Here's the drawing with two shaded views (mm, measured from the low corner). I have some questions. A direction names the side the tool comes from. Give positions to 0.01 mm unless a question says otherwise; leave off trailing zeros. Write each loop counter-clockwise with the first axis right and the second up, starting at its lowest first coordinate (ties: lowest second). Pieces come first, ordered by that corner, then holes.
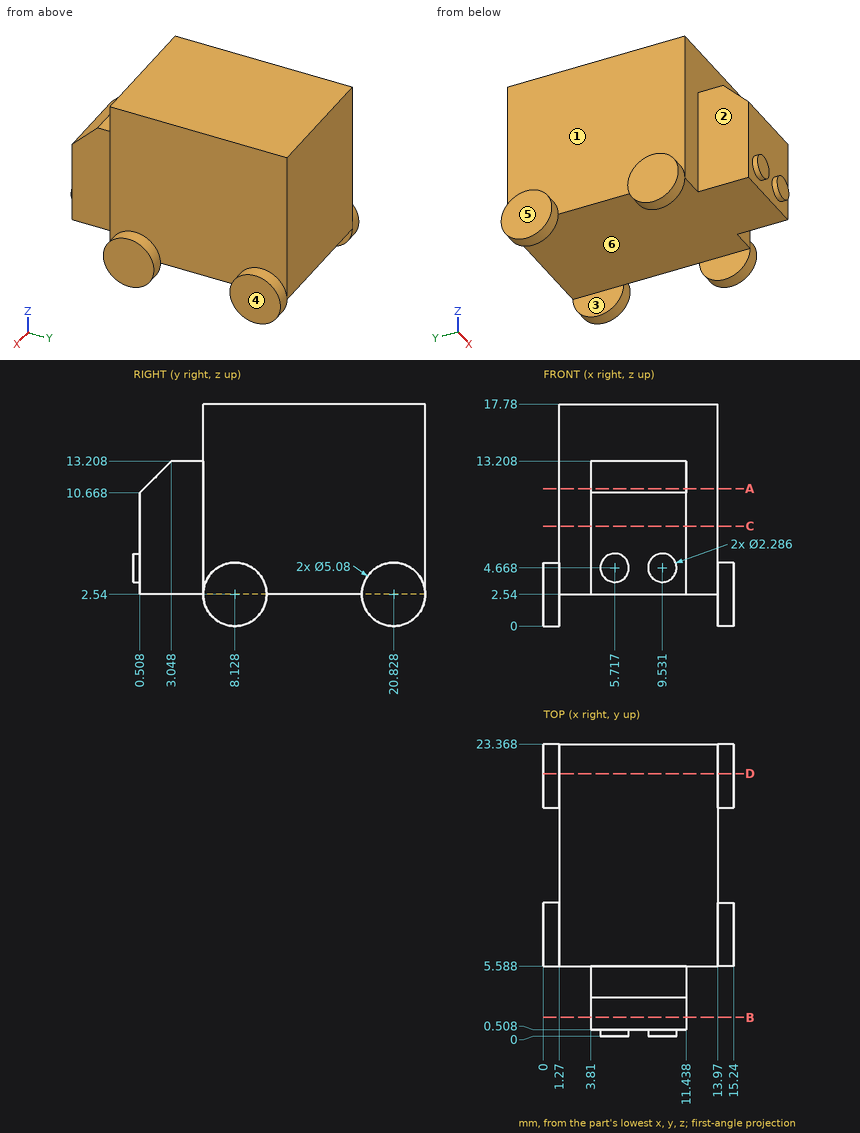
(1) Imagine slicing it at B-B, the plane y = 1.5. Write out the boundary of the cut face in (x, z).
Returned:
outline: (3.81, 2.54) - (11.44, 2.54) - (11.44, 11.66) - (3.81, 11.66) - close
(2) For the marked faces 1, 2 and 3, which set-ups out of +Z, -Z, +X, -X, +Y, -Y let a thin tool reach every point of the face, with its end or its side?
Returned:
face 1: +Z, -X
face 2: +Z, -Z, -X, -Y
face 3: -Z, +Y, -Y
(3) Imagine slicing it at D-D, the plane y = 21. Write out the boundary of the cut face in (x, z) (1 decimal).
Returned:
outline: (0, 0) - (1.3, 0) - (1.3, 2.5) - (14, 2.5) - (14, 0) - (15.2, 0) - (15.2, 5.1) - (14, 5.1) - (14, 17.8) - (1.3, 17.8) - (1.3, 5.1) - (0, 5.1) - close
(4) Imagine slicing it at C-C, the plane z = 8. Write out the boundary of the cut face in (x, y).
Returned:
outline: (1.27, 5.59) - (3.81, 5.59) - (3.81, 0.51) - (11.44, 0.51) - (11.44, 5.59) - (13.97, 5.59) - (13.97, 23.37) - (1.27, 23.37) - close
(5) Imagine slicing it at A-A, the plane z = 11. Write out the boundary of the cut face in (x, y), plus the area to 3 significant figures.
Returned:
outline: (1.27, 5.59) - (3.81, 5.59) - (3.81, 0.84) - (11.44, 0.84) - (11.44, 5.59) - (13.97, 5.59) - (13.97, 23.37) - (1.27, 23.37) - close
area: 262 mm2
(6) If we mould it in two halves opening along X, with no side actions, what happens to the marked faces 4, 5 and 6? For each: +X half, -X half, draft (parallel to the pull), parting line (faces both ways), or undercut.
Returned:
face 4: +X half
face 5: -X half
face 6: undercut
(7) Will these pins go through, and if not, where does the flat tip stop? P1, Ø7.5, axis at y = 10.5, z = 11, coming from the -X side; P2, Ø4, axis at x = 13, z = 8.5, coming from the -Y side; P3, Ø1.5, axis at y = 4, z = 10, coming from the +X side.
Returned:
P1: stops at x = 1.27
P2: stops at y = 0.51
P3: stops at x = 11.44
(8) If I drill on L1, parallel to Z at x = 1.5, y = 19.5; L2, parallel to Y at x = 6.75, z = 3.25; L3, parallel to Y at x = 10.75, z = 16.25, over which ranges is the centre line in solid material (lowest first)?
Returned:
L1: z = 2.54 to 17.78
L2: y = 0.51 to 23.37
L3: y = 5.59 to 23.37
